```python
from build123d import *

# Parameters (mm, degrees)
F0_W     = 40
F0_H     = 40
F0_R     = 3.5
F1_DEPTH = 8
F2_R     = 2.1
F3_DEPTH = 12
F4_R     = 2.1
F5_DEPTH = 12
F6_R     = 9


with BuildPart() as f1:
    # F0 (on Top) → F1 (new body)
    with BuildSketch(Plane.XY):
        Polygon((-30, 0), (-30, 16.25), (-35, 5), (-35, 0), (-35, -5), (-30, -16.25), align=None)
        Polygon((-20, -20), (-20, 20), (-30, 16.25), (-30, 0), (-30, -16.25), align=None)
        Polygon((-26.5094576257, -11.7926480899), (-27.9309422569, -8.5943076697), (-29.3524268881, -5.3959672496), (-25.6971806936, -3.7714133853), (-22.8542114312, -10.1680942257), align=None, mode=Mode.SUBTRACT)
        Polygon((-29.3524268881, 5.3959672496), (-27.9309422569, 8.5943076697), (-26.5094576257, 11.7926480899), (-22.8542114312, 10.1680942257), (-25.6971806936, 3.7714133853), align=None, mode=Mode.SUBTRACT)
        Rectangle(F0_W, F0_H)
        Circle(F0_R, mode=Mode.SUBTRACT)
    extrude(amount=F1_DEPTH)

    # F2 (on face) → F3 (cut)
    with BuildSketch(Plane(origin=(-31.0824742268, 13.8144329897, 0), x_dir=(-0.4061384661, -0.9138115486, 0), z_dir=(-0.9138115486, 0.4061384661, 0))):
        with Locations((3.4902524426, 4)):
            Circle(F2_R)
    extrude(amount=-F3_DEPTH, mode=Mode.SUBTRACT)

    # F4 (on face) → F5 (cut)
    with BuildSketch(Plane(origin=(-31.0824742268, -13.8144329897, 0), x_dir=(0.4061384661, -0.9138115486, 0), z_dir=(-0.9138115486, -0.4061384661, 0))):
        with Locations((-3.4902524426, 4)):
            Circle(F4_R)
    extrude(amount=-F5_DEPTH, mode=Mode.SUBTRACT)

    # F6
    f6_edges = [f1.edges().sort_by_distance(p)[0] for p in [
        (20, -20, 4),
        (20, 20, 4),
        (-20, -20, 4),
        (-30, -16.25, 4),
        (-35, -5, 4),
        (-35, 5, 4),
        (-30, 16.25, 4),
        (-20, 20, 4),
    ]]
    fillet(f6_edges, radius=F6_R)


solid = f1.part
```
Model file for the job. Use its own axes, mm. A direction names the side the tool comes from. Coordinates: 2 decimals unless noted, no trailing zeros. Loops run counter-clockwise (first coordinate to the right, second up) from the corner with the lowest first, then second, coordinate; pieces in that order, holes last. Notation, with made-up numbers: (-24, 35.25) - (30, 35.25) arc R38 cw to (30, 73.25) - close; hole circle Ø9 at (51.5, 31.25). An arc over 180 degrees is marked (long way). Answer as a JSON object with one key per item and string values. Group by question number.
(1) Flat gauge pin, fed straight in: pin 1 (10 mm diameter, centred on x = 5, y = 0.5, fed in from -Z). Where does the tip first touch, or does it go through?
(2) Cut at C-C (x = -24). State how many separate pieces and enclosed holes the cut face has, then the cut area to 3 significant figures.
(3) Two-plate mould, pull along X, no slides. Class faces 1 (the face through (-33.458, 8.47, 3.944)), 2 (the face through (17.434, -17.294, 4.056)), 3 (the face through (-23.308, 9.147, 3.944)), 4 (the face through (-8, 0, 8)): released by +X, released by -X, zero draft, split by the parting line, or undercut.
(4) Cut at B-B (x = 0). Give the cut face in (y, z).
(5) Tool access for faces 5 (the face through (-27.55, -4.595, 3.944)), 6 (the face through (-30.06, 10.04, 1.95)): list every direction of +Z, -Z, +X, -X, +Y, -Y with a clear straight run to the whole face (end or side of a thin tool).
(6) Cut at A-A (y = 0). Give the cut face in (x, z), then the cut area to 3 significant figures.
(7) Probe line 1 along Y through (x, z) = (-30, 2.5); line 2 along Y through (x, z) = (0, 3.5); line 3 along Y through (x, z) = (-28, 6.5). List the from-to ranges inside material, lowest first.
(8) Cut at D-D (y = 16.5). Give the cut face in (x, z).
Geometry says:
{
 "1": {"pin 1": "stops at z = 0"},
 "2": {"separate pieces": "3", "enclosed holes": "0", "area": "225 mm^2"},
 "3": {"face 1": "released by -X", "face 2": "released by +X", "face 3": "undercut", "face 4": "zero draft"},
 "4": {"outline": "(-20, 0) - (-3.5, 0) - (-3.5, 8) - (-20, 8) - close; (3.5, 0) - (20, 0) - (20, 8) - (3.5, 8) - close"},
 "5": {"face 5": "+Z, -Z", "face 6": "none"},
 "6": {"outline": "(-35, 0) - (-3.5, 0) - (-3.5, 8) - (-35, 8) - close; (3.5, 0) - (20, 0) - (20, 8) - (3.5, 8) - close", "area": "384 mm^2"},
 "7": {"line 1": "y = -15.17 to -11.12, -7.91 to 7.91, 11.12 to 15.17", "line 2": "y = -20 to -3.5, 3.5 to 20", "line 3": "y = -16.83 to -8.44, -4.79 to 4.79, 8.44 to 16.83"},
 "8": {"outline": "(-28.5, 0) - (18.12, 0) - (18.12, 8) - (-28.5, 8) - close"}
}
